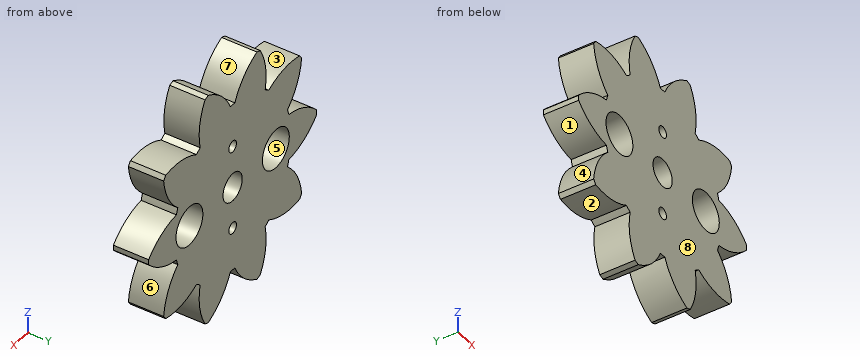
```python
from build123d import *

# Parameters (mm, degrees)
SKETCH1_R           = 17.5
BOSS_EXTRUDE1_DEPTH = 5
CUT_EXTRUDE1_START  = -5
CUT_EXTRUDE1_DEPTH  = 5
CIRPATTERN1_COUNT   = 10
SKETCH3_R           = 2
CUT_EXTRUDE2_DEPTH  = 5
SKETCH4_R           = 0.8
SKETCH4_R_2         = 2.8
CUT_EXTRUDE3_DEPTH  = 5


with BuildPart() as part:
    # Sketch1 → Boss-Extrude1 (new body)
    with BuildSketch(Plane(origin=(0, 0, 0), x_dir=(1, 0, 0), z_dir=(0, 1, 0))):
        with Locations(Location((0, 0, 0), (0, 0, 270))):
            Circle(SKETCH1_R)
    extrude(amount=BOSS_EXTRUDE1_DEPTH)

    # Sketch2 → Cut-Extrude1 (cut)
    with BuildSketch(Plane(origin=(0, 5, 0), x_dir=(1, 0, 0), z_dir=(0, 1, 0)).offset(CUT_EXTRUDE1_START)):
        with BuildLine():
            ThreePointArc((-0.461351562, 12.161707059), (-2.330748839, 14.886662879), (-5.057656399, 16.753211983))
            ThreePointArc((-5.057656399, 16.753211983), (0, 17.5), (5.057656399, 16.753211983))
            ThreePointArc((5.057656399, 16.753211983), (2.330748839, 14.886662879), (0.461351562, 12.161707059))
            ThreePointArc((0.461351562, 12.161707059), (0, 12.170454545), (-0.461351562, 12.161707059))
        make_face()
    cut_extrude1 = extrude(amount=CUT_EXTRUDE1_DEPTH, mode=Mode.SUBTRACT)

    # CirPattern1: Cut-Extrude1 ×10 about axis
    cirpattern1_axis = Axis((0, 0, 0), (0, 1, 0))
    for i in range(1, CIRPATTERN1_COUNT):
        add(cut_extrude1.rotate(cirpattern1_axis, i * 360 / CIRPATTERN1_COUNT), mode=Mode.SUBTRACT)

    # Sketch3 → Cut-Extrude2 (cut)
    with BuildSketch(Plane(origin=(0, 5, 0), x_dir=(1, 0, 0), z_dir=(0, 1, 0))):
        with Locations(Location((0, 0, 0), (0, 0, 270))):
            Circle(SKETCH3_R)
    extrude(amount=-CUT_EXTRUDE2_DEPTH, mode=Mode.SUBTRACT)

    # Sketch4 → Cut-Extrude3 (cut)
    with BuildSketch(Plane(origin=(0, 5, 0), x_dir=(1, 0, 0), z_dir=(0, 1, 0))):
        with Locations(Location((0, 6, 0), (0, 0, 270))):
            Circle(SKETCH4_R)
        with Locations(Location((0, -6, 0), (0, 0, 270))):
            Circle(SKETCH4_R)
        with Locations(Location((-9, 0, 0), (0, 0, 270))):
            Circle(SKETCH4_R_2)
        with Locations(Location((9, 0, 0), (0, 0, 270))):
            Circle(SKETCH4_R_2)
    extrude(amount=-CUT_EXTRUDE3_DEPTH, mode=Mode.SUBTRACT)


solid = part.part
```
Check sheet for the modelled part. Datum: model origin and axes. Units: mm. Face numbers are marked on the shaded views. A direction names the side the tool comes from. Give positions to 0.01 mm unless a question says otherwise; leave off trailing zeros. Write each loop counter-clockwise with the first axis right and the second up, starting at its lowest first coordinate (ties: lowest second). Pieces come first, ordered by that corner, then holes.
Item 1: Cross-section at B-B (z = 14.5). Enter the section's corners in (x, y), and give its area (3 significant figures).
Item 2: Access from +Z, -Z, +X, -X, +Y, -Y to the whole of each face (thin tool, end or side, straight path). Record for the marked faces 4, 5, 6, 7 and 8.
Item 3: Cross-section at D-D (z = 6). Enter the section's corners in (x, y), and give its area (3 significant figures).
Item 4: Cross-section at C-C (y = 2). Count the separate pieces of the cut face and the enclosed holes in it, and give its area (3 significant figures).
Item 5: Draft check along Z on the marked faces 1, 2 and 3. Enter one of: released by +Z, released by -Z, zero draft, split by the parting line, or undercut.
Item 6: Scan lines: L1, parallel to X at y = 3.7, z = 0; L2, parallel to Z at x = 13.5, y = 0.35; L3, parallel to X at y = 2.55, z = 0.5 (1 decimal). Record each from-to range of solid material in increasing order.
Item 7: Cross-section at A-A (x = 0). Enter the section's corners in (y, z).
Item 8: Gauge pin test, flat ends, axial feed: pin 1 (1 mm diameter, centred on x = 0, z = -6, fed in from -Y); pin 2 (12 mm diameter, centred on x = 12.5, z = -1, fed in from -Y); pin 3 (1.5 mm diameter, centred on y = 0.5, z = 6.5, fed in from +X); pin 4 (3 mm diameter, centred on y = 1.5, z = -7.5, fed in from -X). Record the tip position at first contact, or that the pin passes through.
Report:
1. outline: (-6.62, 0) - (-1.97, 0) - (-1.97, 5) - (-6.62, 5) - close; (1.97, 0) - (6.62, 0) - (6.62, 5) - (1.97, 5) - close
1. area: 46.6 mm2
2. face 4: -X, +Y, -Y
2. face 5: +Y, -Y
2. face 6: +X, +Y, -Y
2. face 7: +Z, +Y, -Y
2. face 8: +Z, -Z, +X, -X, -Y
3. outline: (-12.97, 0) - (-0.8, 0) - (-0.8, 5) - (-12.97, 5) - close; (0.8, 0) - (12.97, 0) - (12.97, 5) - (0.8, 5) - close
3. area: 122 mm2
4. separate pieces: 1
4. enclosed holes: 5
4. area: 645 mm2
5. face 1: undercut
5. face 2: released by -Z
5. face 3: released by +Z
6. L1: x = -17.5 to -11.8, -6.2 to -2, 2 to 6.2, 11.8 to 17.5
6. L2: z = -10.66 to -6.94, -2.95 to 2.95, 6.94 to 10.66
6. L3: x = -17.4 to -11.8, -6.2 to -1.9, 1.9 to 6.2, 11.8 to 17.4
7. outline: (0, -12.17) - (5, -12.17) - (5, -6.8) - (0, -6.8) - close; (0, -5.2) - (5, -5.2) - (5, -2) - (0, -2) - close; (0, 2) - (5, 2) - (5, 5.2) - (0, 5.2) - close; (0, 6.8) - (5, 6.8) - (5, 12.17) - (0, 12.17) - close
8. pin 1: passes through
8. pin 2: stops at y = 0
8. pin 3: stops at x = 13.64
8. pin 4: stops at x = -14.21
